Part model, mm, in its own coordinate system. A direction names the side the tool comes from. Give positions to 0.01 mm unless a question says otherwise; leave off trailing zeros. Order: outer loops, then holes, each group sorted by start corner. A loop starts at its lowest first (then second) coordinate and runs counter-clockwise, first axis right, second up. Notation, with made-up numbers: M 3,81.25 L 39,81.25 A6 cw 39,85.25 Z; hole C 4,57.25 d8. An arc over 180 degrees is marked long. Answer as a JSON object with one key per item and string values.
from build123d import *

# Parameters (mm, degrees)
CROQUIS1_W              = 40
CROQUIS1_H              = 3
CROQUIS1_H_2            = 2
CROQUIS1_W_2            = 5
CROQUIS1_H_3            = 8
CROQUIS1_R              = 4
SALIENTE_EXTRUIR1_DEPTH = 10


with BuildPart() as part:
    # Croquis1 → Saliente-Extruir1 (new body)
    with BuildSketch(Plane.XY):
        with BuildLine():
            Line((-25, 10), (-25, 0))
            Line((-25, 0), (25, 0))
            Line((25, 0), (25, 10))
            Line((25, 10), (30, 10))
            Line((30, 10), (30, 0))
            Line((30, 0), (50, 0))
            Line((50, 0), (70, 20.022237637))
            Line((70, 20.022237637), (70, 30.022237637))
            Line((70, 30.022237637), (50, 30.022237637))
            Line((50, 30.022237637), (50, 33.022237637))
            Line((50, 33.022237637), (37.9, 33.022237637))
            ThreePointArc((37.9, 33.022237637), (31.9, 39.022237637), (25.9, 33.022237637))
            Line((25.9, 33.022237637), (-25.9, 33.022237637))
            ThreePointArc((-25.9, 33.022237637), (-31.9, 39.022237637), (-37.9, 33.022237637))
            Line((-37.9, 33.022237637), (-50, 33.022237637))
            Line((-50, 33.022237637), (-50, 30.022237637))
            Line((-50, 30.022237637), (-70, 30.022237637))
            Line((-70, 30.022237637), (-70, 20.022237637))
            Line((-70, 20.022237637), (-50, 0))
            Line((-50, 0), (-30, 0))
            Line((-30, 0), (-30, 10))
            Line((-30, 10), (-25, 10))
        make_face()
        with Locations((0, 11.5)):
            Rectangle(CROQUIS1_W, CROQUIS1_H, mode=Mode.SUBTRACT)
        with Locations((0, 16)):
            Rectangle(CROQUIS1_W, CROQUIS1_H_2, mode=Mode.SUBTRACT)
        with Locations((-64.5, 24.522237637)):
            Rectangle(CROQUIS1_W_2, CROQUIS1_H_3, mode=Mode.SUBTRACT)
        with BuildLine():
            ThreePointArc((-27.9, 33.022237637), (-31.9, 29.022237637), (-35.9, 33.022237637))
            ThreePointArc((-35.9, 33.022237637), (-31.9, 37.022237637), (-27.9, 33.022237637))
        make_face(mode=Mode.SUBTRACT)
        with Locations((0, 21.5)):
            Rectangle(CROQUIS1_W, CROQUIS1_H, mode=Mode.SUBTRACT)
        with Locations((0, 27)):
            Rectangle(CROQUIS1_W, CROQUIS1_H_2, mode=Mode.SUBTRACT)
        with Locations((64.5, 24.522237637)):
            Rectangle(CROQUIS1_W_2, CROQUIS1_H_3, mode=Mode.SUBTRACT)
        with Locations((31.9, 33.022237637)):
            Circle(CROQUIS1_R, mode=Mode.SUBTRACT)
    extrude(amount=SALIENTE_EXTRUIR1_DEPTH)


solid = part.part
1. Cut at D-D on z = 2. State how many separate pieces and enclosed holes the cut face has, plus the area to 3 significant figures.
Worked answers:
{"separate pieces": "1", "enclosed holes": "8", "area": "3,540 mm^2"}
2. Pin check, flat tips, straight feed: P1, Ø3.5, axis at y = 11, z = 5.5, coming from the +X side; P2, Ø3, axis at x = 38, z = 3, coming from the +Y side; P3, Ø3, axis at y = 4, z = 3, coming from the +X side. Stop position of each tip, or through.
Worked answers:
{"P1": "stops at x = 62.74", "P2": "stops at y = 36.87", "P3": "stops at x = 55.49"}
3. Probe line 1 along Y through (x, z) = (-9.5, 4.25); line 2 along Y through (x, z) = (31.9, 4.25); line 3 along X through (y, z) = (6, 6.25). List the from-to ranges inside material, lowest first.
Worked answers:
{"line 1": "y = 0 to 10, 13 to 15, 17 to 20, 23 to 26, 28 to 33.02", "line 2": "y = 0 to 29.02, 37.02 to 39.02", "line 3": "x = -55.99 to -30, -25 to 25, 30 to 55.99"}
4. Cut at C-C on y = 35.5. Give the cut face in (x, z).
Worked answers:
{"outline": "M -37.36,0 L -35.04,0 L -35.04,10 L -37.36,10 Z; M -28.76,0 L -26.44,0 L -26.44,10 L -28.76,10 Z; M 26.44,0 L 28.76,0 L 28.76,10 L 26.44,10 Z; M 35.04,0 L 37.36,0 L 37.36,10 L 35.04,10 Z"}
5. Which spindle directions (+Z, -Z, +X, -X, +Y, -Y) get a long thin tool onto all of the face, cutting with end or side? Do faces 5 (the flat face through (-44, 33.022, 5)), 6 (the flat face through (0, 33.022, 5)), 7 (the flat face through (-67, 24, 5)), 8 (the flat face through (-1, 19.8, 0)), 9 (the flat face through (44, 33.022, 5)). Say none if no direction does.
Worked answers:
{"face 5": "+Z, -Z, -X, +Y", "face 6": "+Z, -Z, +Y", "face 7": "+Z, -Z", "face 8": "-Z, +X, -X, +Y, -Y", "face 9": "+Z, -Z, +X, +Y"}
6. Cut at B-B on x = 31.9. Give the cut face in (y, z).
Worked answers:
{"outline": "M 0,0 L 29.02,0 L 29.02,10 L 0,10 Z; M 37.02,0 L 39.02,0 L 39.02,10 L 37.02,10 Z"}
7. Cut at A-A on x = -18. Give the cut face in (y, z).
Worked answers:
{"outline": "M 0,0 L 10,0 L 10,10 L 0,10 Z; M 13,0 L 15,0 L 15,10 L 13,10 Z; M 17,0 L 20,0 L 20,10 L 17,10 Z; M 23,0 L 26,0 L 26,10 L 23,10 Z; M 28,0 L 33.02,0 L 33.02,10 L 28,10 Z"}
8. Two-plate mould, pull along X, no slides. Class faces 1 (the cylindrical face through (32.03, 39.02, 4.93)), 2 (the flat face through (-70, 25, 5)), 3 (the flat face through (64, 28.522, 5)), 4 (the flat face through (40, 0, 5)): +X half, -X half, draft (parallel to the pull), parting line (faces both ways), or undercut.
Worked answers:
{"face 1": "undercut", "face 2": "-X half", "face 3": "undercut", "face 4": "draft"}
